```python
from build123d import *

# Parameters (mm, degrees)
SKETCH_W      = 60
SKETCH_H      = 60
PAD_DEPTH     = 10
SKETCH001_R   = 20
SKETCH001_R_2 = 15
PAD001_DEPTH  = 20


with BuildPart() as part:
    # Sketch → Pad (new body)
    with BuildSketch(Plane.XZ):
        Rectangle(SKETCH_W, SKETCH_H)
    extrude(amount=-PAD_DEPTH)

    # Sketch001 (on Face6 of Pad) → Pad001 (join)
    with BuildSketch(Plane(origin=(0, 10, 0), x_dir=(1, 0, 0), z_dir=(0, 1, 0))):
        Circle(SKETCH001_R)
        Circle(SKETCH001_R_2, mode=Mode.SUBTRACT)
    extrude(amount=PAD001_DEPTH)


solid = part.part
```
Input: part model. Units: mm. Frame: model coordinates. A direction names the side the tool comes from. Give positions to 0.01 mm unless a question says otherwise; leave off trailing zeros. Order: outer loops, then holes, each group sorted by start corner. A loop starts at its lowest first (then second) coordinate and runs counter-clockwise, first axis right, second up.
1. Mould query, pull axis Z, two halves, no side actions, for faces 1 (the flat face through (0, 0, 0)), 2 (the flat face through (0, 5, -30)), 3 (the cylindrical face through (-14.985, 19.86, -0.66)), 4 (the cylindrical face through (-4.336, 19.86, 19.524)). Classes: released by +Z, released by -Z, zero draft, split by the parting line, or undercut.
Derived:
face 1: zero draft
face 2: released by -Z
face 3: undercut
face 4: split by the parting line
2. Material intervals for L1, parallel to Z at x = 0, y = 16; L2, parallel to Y at x = 10.5, z = -6.5, sorted ascending.
Derived:
L1: z = -20 to -15, 15 to 20
L2: y = 0 to 10
3. Pin query (flat end, axial travel): pin 1 (2 mm diameter, centred on y = 16, z = 0.5, fed in from -X); pin 2 (1 mm diameter, centred on x = -15.5, z = 14.5, fed in from +Y); pin 3 (4 mm diameter, centred on x = 19, y = 15.5, fed in from +Z). Return the tip coordinate at first contact, or that it passes through.
Derived:
pin 1: stops at x = -20
pin 2: stops at y = 10
pin 3: stops at z = 10.54
4. Reachability of faces 5 (the flat face through (-30, 5, 0)), 6 (the flat face through (0, 10, 0)) from +Z, -Z, +X, -X, +Y, -Y: full face, straight path, thin tool, end or side. Return the list, or none.
Derived:
face 5: +Z, -Z, -X, +Y, -Y
face 6: +Y
5. Section A-A on z = 0. Return the cut outline in (x, y).
Derived:
outline: (-30, 0) - (30, 0) - (30, 10) - (20, 10) - (20, 30) - (15, 30) - (15, 10) - (-15, 10) - (-15, 30) - (-20, 30) - (-20, 10) - (-30, 10) - close
6. Section D-D on x = 0. Return the cut outline in (y, z), and give its area (3 significant figures).
Derived:
outline: (0, -30) - (10, -30) - (10, -20) - (30, -20) - (30, -15) - (10, -15) - (10, 15) - (30, 15) - (30, 20) - (10, 20) - (10, 30) - (0, 30) - close
area: 800 mm2
7. Section C-C on y = 21.5. Return the cut outline in (x, z).
Derived:
outline: circle Ø40 at (0, 0); hole circle Ø30 at (0, 0)
8. Section B-B on x = -16. Return the cut outline in (y, z).
Derived:
outline: (0, -30) - (10, -30) - (10, -12) - (30, -12) - (30, 12) - (10, 12) - (10, 30) - (0, 30) - close
